Model file for the job. Use its own axes, mm. Coordinates: 2 decimals unless noted, no trailing zeros. Order: outer loops, then holes, each group sorted by start corner. A loop starts at its lowest first (then second) coordinate and runs counter-clockwise, first axis right, second up. Notation, with made-up numbers: (-5, -36) -> (32, -36) arc R19 ccw to (32, 0) -> close; hole circle Ø3 at (27, 61). An arc over 180 degrees is marked (long way). Write item = value, one per line. Start each with the question number.
Q1. Cut at A-A, the plane y = 10.5. List the corners of the cut face in (x, z), plus the area to 3 significant figures.
Q2. Mould opens along Y. For faces 1 (the face through (-29, 9, 0)), 2 (the face through (-23.254, 24.436, 1.521)), 3 (the face through (-23.3, 3.9, 1.5)), 4 (the face through (-36.966, 15.132, 1.479)) say: +Y half, -Y half, draft (parallel to the pull), parting line (faces both ways), or undercut.
Q3. Flat gauge pin, fed straight in: pin 1 (10 mm diameter, centred on x = -27.5, y = 15, fed in from +Z). Where does the tip first touch, or does it go through?
Q4. Cut at B-B, the plane x = -36. List the corners of the cut face in (y, z), plus the area to 3 significant figures.
Q5. Cut at C-C, the plane z = 1.15. List the corners of the cut face in (x, y), plus the area to 3 significant figures.
Q6. Cut at D-D, the plane x = -23.5. List the corners of the cut face in (y, z).
Q7. Wall check: line 1 (X direction, y = 15, z = 2.4); line 2 (Y direction, x = -33.5, z = 0.35); line 3 (X direction, y = 18, z = 2.4). Give the ranges that are in metal, low to high. Write a range as from..to.
from build123d import *

# Parameters (mm, degrees)
F0_W     = 18.437991
F0_H     = 23.499398
F1_DEPTH = 3
F2_R     = 5
F3_R     = 5.946715
F4_DEPTH = 3


with BuildPart() as f1:
    # F0 (on Top) → F1 (new body)
    with BuildSketch(Plane.XY):
        with Locations((-31.047585, 14.190282)):
            Rectangle(F0_W, F0_H)
    extrude(amount=F1_DEPTH)

    # F2
    f2_edges = [f1.edges().sort_by_distance(p)[0] for p in [
        (-40.266581, 25.939981, 1.5),
        (-21.82859, 25.939981, 1.5),
        (-21.82859, 2.440583, 1.5),
        (-40.266581, 2.440583, 1.5),
    ]]
    fillet(f2_edges, radius=F2_R)

    # F3 (on Top) → F4 (cut)
    with BuildSketch(Plane.XY):
        with Locations((-31.025298, 14.870087)):
            Circle(F3_R)
    extrude(amount=F4_DEPTH, mode=Mode.SUBTRACT)


solid = f1.part
Here are the results:
q1.outline = (-40.27, 0) -> (-35.06, 0) -> (-35.06, 3) -> (-40.27, 3) -> close; (-26.99, 0) -> (-21.83, 0) -> (-21.83, 3) -> (-26.99, 3) -> close
q1.area = 31.1 mm²
q2.face_1 = draft
q2.face_2 = +Y half
q2.face_3 = -Y half
q2.face_4 = undercut
q3.pin_1 = 3
q4.outline = (2.49, 0) -> (11.61, 0) -> (11.61, 3) -> (2.49, 3) -> close; (18.13, 0) -> (25.89, 0) -> (25.89, 3) -> (18.13, 3) -> close
q4.area = 50.6 mm²
q5.outline = (-40.27, 7.44) arc R5 ccw to (-35.27, 2.44) -> (-26.83, 2.44) arc R5 ccw to (-21.83, 7.44) -> (-21.83, 20.94) arc R5 ccw to (-26.83, 25.94) -> (-35.27, 25.94) arc R5 ccw to (-40.27, 20.94) -> close; hole circle Ø11.89 at (-31.03, 14.87)
q5.area = 301 mm²
q6.outline = (3.71, 0) -> (24.67, 0) -> (24.67, 3) -> (3.71, 3) -> close
q7.line_1 = -40.27..-36.97, -25.08..-21.83
q7.line_2 = 2.44..9.46, 20.28..25.94
q7.line_3 = -40.27..-36.08, -25.97..-21.83
